Input: dimensioned drawing with shaded views. Units: mm. Origin: part minimum x, y, z. A direction names the side the tool comes from. Give positions to 0.01 mm unless a question says otherwise; leave off trailing zeros. Loops run counter-clockwise (first coordinate to the right, second up) from the corner with the lowest first, then second, coordinate; pieces in that order, holes last. Notation, with made-up numbers: M 67.5,62 L 115.5,62 A18 cw 115.5,91 Z; hole C 10.5,-33.75 d7. An arc over 180 degrees is marked long. Answer in a Markdown table with one row per item.
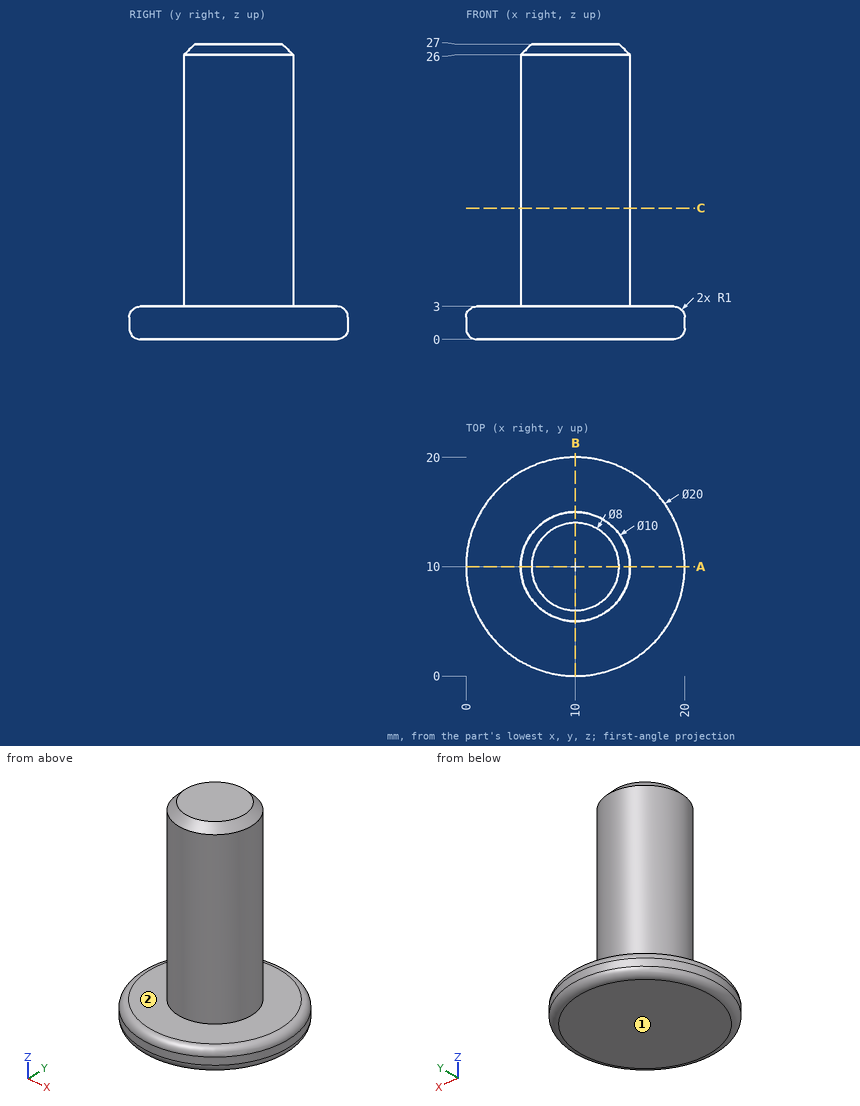
Q1. Reachability of the marked faces 1 and 2 from +Z, -Z, +X, -X, +Y, -Y: full face, straight path, thin tool, end or side. Return the list, or none.
Values follow:
| item | result |
|---|---|
| face 1 | -Z, +X, -X, +Y, -Y |
| face 2 | +Z |
Q2. Ray query, probe 1 along Z at (x, y) = (16.25, 13.75); probe 2 along X at (y, z) = (10, 19.5); probe 3 along X at (y, z) = (6.75, 12.75). Return the intervals inside material, ascending. Write a range as from..to.
Values follow:
| item | result |
|---|---|
| probe 1 | 0..3 |
| probe 2 | 5..15 |
| probe 3 | 6.2..13.8 |
Q3. Section query A-A (y = 10). Output: boundary loops of the cut face in (x, z), plus the area to 3 significant figures.
Values follow:
| item | result |
|---|---|
| outline | M 0,1 A1 ccw 1,0 L 19,0 A1 ccw 20,1 L 20,2 A1 ccw 19,3 L 15,3 L 15,26 L 14,27 L 6,27 L 5,26 L 5,3 L 1,3 A1 ccw 0,2 Z |
| area | 298 mm^2 |
Q4. Contact query for flat-ended pins moving along their axis: pin 1 Ø5 at (x, z) = (9, 13.5) entering from +Y; pin 2 Ø2 at (x, y) = (7, 16) entering from +Z; pin 3 Ø4 at (x, z) = (15, 13) entering from -Y. Output: stop coordinate, or through.
Values follow:
| item | result |
|---|---|
| pin 1 | y = 15 |
| pin 2 | z = 3 |
| pin 3 | y = 6 |
Q5. Section query C-C (z = 12). Output: boundary loops of the cut face in (x, y), plus the area to 3 significant figures.
Values follow:
| item | result |
|---|---|
| outline | C 10,10 d10 |
| area | 78.5 mm^2 |
